The listing builds one solid part. Answer for the finished solid, in the listing's coordinates (mm). Coordinates: 2 decimals unless noted, no trailing zeros. Order: outer loops, then holes, each group sorted by start corner. A loop starts at its lowest first (then second) coordinate and runs counter-clockwise, first axis right, second up. Notation, with made-up numbers: (-31.75, -15.5) -> (-11.75, -15.5) arc R23 ccw to (-11.75, 13.5) -> close; hole circle Ø4 at (44.25, -26.5). An arc over 180 degrees is marked (long way). One line per question, with ' | ' between items.
from build123d import *

# Parameters (mm, degrees)
BOSS_EXTRUDE2_START = 1
SKETCH3_W           = 24
SKETCH3_H           = 24
BOSS_EXTRUDE2_DEPTH = 39.5
FILLET1_R           = 10


with BuildPart() as part:
    # Sketch1 → Revolve1 (revolve)
    with BuildSketch(Plane(origin=(0, 0, 0), x_dir=(0, 0, -1), z_dir=(1, 0, 0))):
        Polygon((0, 0), (10.5, 10), (10.5, 38.857142857), (11.25, 40.5), (11.25, 44.5), (0, 44.5), align=None)
    revolve(axis=Axis((0, 0, 0), (0, 1, 0)))


with BuildPart() as body_2:
    # Sketch3 → Boss-Extrude2 (new body)
    with BuildSketch(Plane(origin=(0, 0, 0), x_dir=(1, 0, 0), z_dir=(0, 1, 0)).offset(BOSS_EXTRUDE2_START)):
        Rectangle(SKETCH3_W, SKETCH3_H)
    extrude(amount=BOSS_EXTRUDE2_DEPTH)

    # Combine1: cut part
    add(part.part, mode=Mode.SUBTRACT)

    # Fillet1
    fillet1_edges = [body_2.edges().sort_by_distance(p)[0] for p in [
        (12, 20.75, 12),
        (-12, 20.75, 12),
        (-12, 20.75, -12),
        (12, 20.75, -12),
    ]]
    fillet(fillet1_edges, radius=FILLET1_R)


solid = body_2.part
Item 1: Section C-C, the plane z = 0 is taken. Give the vertices of the cut face in (x, y), plus the area to 3 significant figures.
Computed values:
outline: (-12, 1) -> (-1.05, 1) -> (-10.5, 10) -> (-10.5, 38.86) -> (-11.25, 40.5) -> (-12, 40.5) -> close; (1.05, 1) -> (12, 1) -> (12, 40.5) -> (11.25, 40.5) -> (10.5, 38.86) -> (10.5, 10) -> close | area: 202 mm^2
Item 2: Section B-B, the plane y = 30 is taken. Give the vertices of the cut face in (x, z), plus the area to 3 significant figures.
Computed values:
outline: (-12, -2) arc R10 ccw to (-2, -12) -> (2, -12) arc R10 ccw to (12, -2) -> (12, 2) arc R10 ccw to (2, 12) -> (-2, 12) arc R10 ccw to (-12, 2) -> close; hole circle Ø21 at (0, 0) | area: 144 mm^2
Item 3: Each of these flat-tipped pins is pushed along its axis until it touches: pin 1 Ø5 at (x, y) = (6.5, 36.5) entering from -Z; pin 2 Ø1.5 at (x, y) = (-6, 31.5) entering from +Z; pin 3 Ø1 at (y, z) = (16.5, 3.5) entering from -X. Where does it stop, or does it pass through?
Computed values:
pin 1: stops at z = -11.8 | pin 2: stops at z = 11.46 | pin 3: stops at x = -11.95
Item 4: Section A-A, the plane x = 0 is taken. Give the vertices of the cut face in (y, z).
Computed values:
outline: (1, -12) -> (40.5, -12) -> (40.5, -11.25) -> (38.86, -10.5) -> (10, -10.5) -> (1, -1.05) -> close; (1, 1.05) -> (10, 10.5) -> (38.86, 10.5) -> (40.5, 11.25) -> (40.5, 12) -> (1, 12) -> close
Item 5: Find the intervals of material crossed by L1, parallel to Z at x = 0, y = 20.5; L2, parallel to X at y = 28, z = -4.25, in increasing order.
Computed values:
L1: z = -12 to -10.5, 10.5 to 12 | L2: x = -11.74 to -9.6, 9.6 to 11.74
Item 6: Section D-D, the plane y = 7.5 is taken. Give the vertices of the cut face in (x, z) (3 decimals).
Computed values:
outline: (-12, -2) arc R10 ccw to (-2, -12) -> (2, -12) arc R10 ccw to (12, -2) -> (12, 2) arc R10 ccw to (2, 12) -> (-2, 12) arc R10 ccw to (-12, 2) -> close; hole circle Ø15.75 at (0, 0)
Item 7: Determine the mould class of faces 1 (the face through (0, 20, -12)), 2 (the face through (8.99, 21.03, 9.15)), 3 (the face through (-3.2, 24.6, -10)) for opening direction X: pulls with the +X half, pulls with the -X half, needs draft (parallel to the pull), parting line crosses it, or undercut.
Computed values:
face 1: needs draft | face 2: pulls with the +X half | face 3: undercut
